Autodesk Inventor part; units mm, degrees
ref_plane "РабПлоскость1" through (26.2, 50, 3) normal (0, 1, 0) x (1, 0, 0)
ref_plane "YZ Plane" through (0, 0, 0) normal (1, 0, 0) x (0, 1, 0)
ref_plane "XZ Plane" through (0, 0, 0) normal (0, 1, 0) x (-1, 0, 0)
sketch "Эскиз1" plane through (0, 0, 0) normal (0, 0, 1) x (1, 0, 0)
  line L0 (0, 0) -> (26.2, 0)
  line L1 (26.2, 0) -> (26.2, 100)
  line L2 (26.2, 100) -> (0, 100)
  line L3 (0, 100) -> (0, 0)
  dimension "d0" = 26.2
  dimension "d1" = 100
extrude "Выдавливание1" add sketch "Эскиз1" along normal blind 3
sketch "Эскиз2" plane through (0, 0, 3) normal (0, 0, 1) x (1, 0, 0)
  line L0 (0, 0) -> (26.2, 0)
  line L1 (13.1, 0) -> (13.1, 5)
  circle A0 centre (13.1, 5) radius 2
  dimension "d4" = 5
  dimension "d5" = 4
extrude "Выдавливание2" cut sketch "Эскиз2" against normal blind 3
pattern_linear "Прямоуг.массив1" count 3 spacing 8 along (1, 0, 0) of "Выдавливание2" first direction both ways yes
sketch "Эскиз3" plane through (0, 0, 3) normal (0, 0, 1) x (1, 0, 0)
  line L0 (26.2, 0) -> (26.2, 100)
  line L1 (26.2, 28.1365) -> (26.2, 15.0365)
  line L2 (26.2, 28.1365) -> (13.1, 28.1365)
  circle A0 centre (13.1, 28.1365) radius 1.5
  point P0 (0, 0)
  dimension "d12" = 13.1
  dimension "d13" = 3
extrude "Выдавливание3" cut sketch "Эскиз3" against normal blind 3
pattern_linear "Прямоуг.массив2" count 3 spacing 25 along (0, 1, 0) of "Выдавливание3"
ref_plane "РабПлоскость1" through (26.2, 50, 3) normal (0, 1, 0) x (1, 0, 0)
mirror "Зеркальное отражение1" about plane through (26.2, 50, 3) normal (0, 1, 0) of "Выдавливание2", "Прямоуг.массив1"
properties part number "000.405 - Рычаг" material "Пластик АБС"
Could you check a few things on this model? Use its own coordinates, in mm. Coordinates: 2 decimals unless noted, no trailing zeros. Order: outer loops, then holes, each group sorted by start corner. A loop starts at its lowest first (then second) coordinate and runs counter-clockwise, first axis right, second up.
Q1. Suppose I cut it at C-C on y = 5. Please give me the cut outline in (x, z), and give its area (3 significant figures).
Q2. Suppose I cut it at D-D on z = 1.65. Give the number of separate pieces and of enclosed holes in the cut face, and give its area (3 significant figures).
Q3. Suppose I cut it at B-B on x = 5.1. Please give me the cut outline in (y, z).
Q4. Please list where these lines run through material, in increasing order: L1, parallel to Y at x = 21.25, z = 2.7; L2, parallel to X at y = 5, z = 1.15; L3, parallel to Y at x = 13.1, z = 1.1.
Q5. Will this pin go through, and if not, where does the flat tip stop? pin 1 (2.5 mm diameter, centred on x = 5.1, y = 5, fed in from -Z).
Q6. Suppose I cut it at A-A on x = 13.1. Please give me the cut outline in (y, z).
Q7. Thinking about a two-plate mould opening in Y: for faces 1 (the flat face through (26.2, 49, 1)), 2 (the flat face through (13, 100, 1)), 3 (the cylindrical face through (7.008, 5.601, 1.521)), which applies, released by +Y, released by -Y, zero draft, split by the parting line, or undercut?
Answer:
1. outline: (0, 0) - (3.1, 0) - (3.1, 3) - (0, 3) - close; (7.1, 0) - (11.1, 0) - (11.1, 3) - (7.1, 3) - close; (15.1, 0) - (19.1, 0) - (19.1, 3) - (15.1, 3) - close; (23.1, 0) - (26.2, 0) - (26.2, 3) - (23.1, 3) - close
1. area: 42.6 mm2
2. separate pieces: 1
2. enclosed holes: 9
2. area: 2,520 mm2
3. outline: (0, 0) - (3, 0) - (3, 3) - (0, 3) - close; (7, 0) - (93, 0) - (93, 3) - (7, 3) - close; (97, 0) - (100, 0) - (100, 3) - (97, 3) - close
4. L1: y = 0 to 3.01, 6.99 to 93.01, 96.99 to 100
4. L2: x = 0 to 3.1, 7.1 to 11.1, 15.1 to 19.1, 23.1 to 26.2
4. L3: y = 0 to 3, 7 to 26.64, 29.64 to 51.64, 54.64 to 76.64, 79.64 to 93, 97 to 100
5. pin 1: passes through
6. outline: (0, 0) - (3, 0) - (3, 3) - (0, 3) - close; (7, 0) - (26.64, 0) - (26.64, 3) - (7, 3) - close; (29.64, 0) - (51.64, 0) - (51.64, 3) - (29.64, 3) - close; (54.64, 0) - (76.64, 0) - (76.64, 3) - (54.64, 3) - close; (79.64, 0) - (93, 0) - (93, 3) - (79.64, 3) - close; (97, 0) - (100, 0) - (100, 3) - (97, 3) - close
7. face 1: zero draft
7. face 2: released by +Y
7. face 3: undercut
